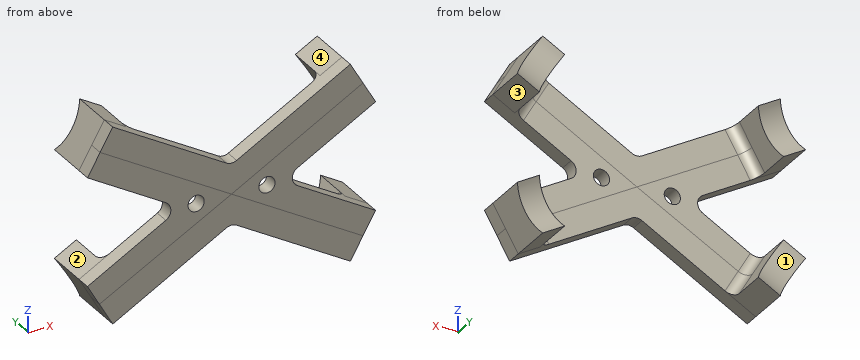
Autodesk Inventor part; units mm, degrees
ref_plane "YZ Plane" through (0, 0, 0) normal (1, 0, 0) x (0, 1, 0)
ref_plane "XZ Plane" through (0, 0, 0) normal (0, 1, 0) x (-1, 0, 0)
ref_plane "XY Plane" through (0, 0, 0) normal (0, 0, 1) x (1, 0, 0)
sketch "Sketch1" plane through (0, 0, 0) normal (0, 1, 0) x (-1, 0, 0)
  arc A0 (-1, 6.3509) -> (1, 6.3509) centre (0, 8.0829) ccw
  arc A1 (-12.9998, -1.7321) -> (-12.9998, 1.7321) centre (-13.9998, 0) ccw
  arc A2 (1, -6.3509) -> (-1, -6.3509) centre (0, -8.0829) ccw
  arc A3 (13, 1.7321) -> (13, -1.7321) centre (14, 0) ccw
  circle A4 centre (7, 0) radius 1.6
  circle A5 centre (-7, 0) radius 1.6
  line L0 (0, 0) -> (26.1212, -14.7541)
  line L1 (0, 0) -> (25.9808, 15)
  line L2 (0, 0) -> (30, 0) construction
  line L3 (0, 0) -> (-25.9808, -15)
  line L4 (0, 0) -> (-25.9808, 15)
  line L5 (0, 0) -> (30, 0) construction
  line L6 (25.9808, 15) -> (28.4808, 10.6699)
  line L7 (25.9808, 15) -> (23.4808, 19.3301)
  line L8 (1, 6.3509) -> (23.4808, 19.3301)
  line L9 (28.4808, 10.6699) -> (13, 1.7321)
  line L10 (13, -1.7321) -> (28.4808, -10.6699)
  line L11 (28.4808, -10.6699) -> (23.4808, -19.3301)
  line L12 (23.4808, -19.3301) -> (1, -6.3509)
  line L13 (-1, -6.3509) -> (-23.4808, -19.3301)
  line L14 (-23.4808, -19.3301) -> (-28.4807, -10.6699)
  line L15 (-28.4807, -10.6699) -> (-12.9998, -1.7321)
  line L16 (-12.9998, 1.7321) -> (-28.4807, 10.6699)
  line L17 (-28.4807, 10.6699) -> (-23.4808, 19.3301)
  line L18 (-23.4808, 19.3301) -> (-1, 6.3509)
  dimension "d0" = 3.2
  dimension "d1" = 30
  dimension "d2" = 30
  dimension "d3" = 30
  dimension "d4" = 30
  dimension "d5" = 30
  dimension "d6" = 150
extrude "Extrusion1" add sketch "Sketch1" along normal blind 3
sketch "Sketch2" plane through (0, 3, 0) normal (0, 1, 0) x (1, 0, 0)
  line L0 (-23.4808, -19.3301) -> (-28.4808, -10.6699)
  line L1 (-28.4808, -10.6699) -> (-24.1506, -8.1699)
  line L2 (-24.1506, -8.1699) -> (-19.1506, -16.8301)
  line L3 (-19.1506, -16.8301) -> (-23.4808, -19.3301)
  line L4 (-28.4808, -10.6699) -> (-23.4808, -19.3301)
  line L5 (-23.4808, 19.3301) -> (-28.4808, 10.6699)
  line L6 (-28.4808, 10.6699) -> (-24.1506, 8.1699)
  line L7 (-24.1506, 8.1699) -> (-19.1506, 16.8301)
  line L8 (-19.1506, 16.8301) -> (-23.4808, 19.3301)
  line L9 (-1, 6.3509) -> (-23.4808, 19.3301)
  line L10 (28.4807, 10.6699) -> (23.4808, 19.3301)
  line L11 (23.4808, 19.3301) -> (19.1506, 16.8301)
  line L12 (19.1506, 16.8301) -> (24.1506, 8.1699)
  line L13 (24.1506, 8.1699) -> (28.4807, 10.6699)
  line L14 (28.4807, -10.6699) -> (23.4808, -19.3301)
  line L15 (23.4808, -19.3301) -> (19.1506, -16.8301)
  line L16 (19.1506, -16.8301) -> (24.1506, -8.1699)
  line L17 (24.1506, -8.1699) -> (28.4807, -10.6699)
  line L18 (23.4808, -19.3301) -> (28.4807, -10.6699)
  point P0 (0, 0)
  dimension "d9" = 5
  dimension "d10" = 5
  dimension "d11" = 5
  dimension "d12" = 5
extrude "Extrusion2" add sketch "Sketch2" along normal blind 15
fillet "Fillet1" radius 2 4 edges at (-21.6506, 3, 12.5) (-21.6506, 3, -12.5) (21.6506, 3, -12.5) (21.6506, 3, 12.5)
sketch "Sketch3" plane through (-19.1506, 5, -16.8301) normal (0.866, 0, 0.5) x (0.5, 0, -0.866)
  line L0 (-10, 13) -> (0, 13)
  circle A0 centre (-5, 13) radius 8
  point P0 (-5, -5)
  dimension "d16" = 16
extrude "Extrusion3" cut sketch "Sketch3" against normal blind 13
sketch "Sketch4" plane through (23.4808, 0, -19.3301) normal (0.866, 0, -0.5) x (-0.5, 0, -0.866)
  line L0 (0, 18) -> (-9.9999, 18)
  circle A0 centre (-5, 18) radius 8
  point P0 (-5, 0)
  dimension "d19" = 16
extrude "Extrusion4" cut sketch "Sketch4" against normal blind 13
sketch "Sketch5" plane through (28.4807, 0, 10.6699) normal (0.866, 0, 0.5) x (0.5, 0, -0.866)
  line L0 (-9.9999, 18) -> (0, 18)
  circle A0 centre (-5, 18) radius 8
  point P0 (-4.9999, 0)
  dimension "d22" = 16
extrude "Extrusion5" cut sketch "Sketch5" against normal blind 10
sketch "Sketch6" plane through (-23.4808, 0, 19.3301) normal (-0.866, 0, 0.5) x (0.5, 0, 0.866)
  line L0 (0, 18) -> (-10, 18)
  circle A0 centre (-5, 18) radius 8
  point P0 (-5, 0)
  dimension "d25" = 16
extrude "Extrusion6" cut sketch "Sketch6" against normal blind 10
properties part number "Motor Support" material "ABS Plastic"
Check sheet for the modelled part. Datum: model origin and axes. Units: mm. Face numbers are marked on the shaded views. Round coordinates to 2 decimals unless told otherwise and drop trailing zeros. Write each loop counter-clockwise with the first axis right and the second up, starting at its lowest first coordinate (ties: lowest second). Pieces come first, ordered by that corner, then holes. Notation, with made-up numbers: (60.25, 9.5) -> (97.25, 9.5) arc R32 cw to (97.25, 46.5) -> close; hole circle Ø3 at (-33, -16.75). An arc over 180 degrees is marked (long way). Put each result on its own line as item: value.
(1) Sectioned sample at B-B (y = 2). Enter the section's corners in (x, z).
Values found:
outline: (-28.48, -10.67) -> (-23.48, -19.33) -> (-1, -6.35) arc R2 cw to (1, -6.35) -> (23.48, -19.33) -> (28.48, -10.67) -> (13, -1.73) arc R2 cw to (13, 1.73) -> (28.48, 10.67) -> (23.48, 19.33) -> (1, 6.35) arc R2 cw to (-1, 6.35) -> (-23.48, 19.33) -> (-28.48, 10.67) -> (-13, 1.73) arc R2 cw to (-13, -1.73) -> close; hole circle Ø3.2 at (-7, 0); hole circle Ø3.2 at (7, 0)
(2) Sectioned sample at D-D (z = 1). Enter the section's corners in (x, y).
Values found:
outline: (-12.27, 0) -> (-8.25, 0) -> (-8.25, 3) -> (-12.27, 3) -> close; (-5.75, 0) -> (5.75, 0) -> (5.75, 3) -> (-5.75, 3) -> close; (8.25, 0) -> (12.27, 0) -> (12.27, 3) -> (8.25, 3) -> close
(3) Material ranges on line 1 (X direction, y = 2, z = 0.5); line 2 (Y direction, x = -13, z = -2.5); line 3 (X direction, y = 1.5, z = -14), recorded low to high.
Values found:
line 1: x = -12.06 to -8.52, -5.48 to 5.48, 8.52 to 12.06
line 2: y = 0 to 3
line 3: x = -26.56 to -14.25, 14.25 to 26.56
(4) Go/stop test with flat-tipped pins: pin 1 Ø4.5 at (x, z) = (2, 8.5) entering from +Y; pin 2 Ø1 at (x, z) = (-20, 12.5) entering from +Y; pin 3 Ø6 at (x, y) = (-12.5, 2) entering from +Z. Record where each tip stops, or that it passes through.
Values found:
pin 1: stops at y = 3
pin 2: stops at y = 3.31
pin 3: stops at z = 14.72
(5) Sectioned sample at C-C (x = 7). Enter the section's corners in (y, z).
Values found:
outline: (0, -9.81) -> (3, -9.81) -> (3, -1.6) -> (0, -1.6) -> close; (0, 1.6) -> (3, 1.6) -> (3, 9.81) -> (0, 9.81) -> close
(6) Sectioned sample at A-A (y = 6.25). Enter the section's corners in (x, z), plus the area to 3 significant figures.
Values found:
outline: (-28.48, -10.67) -> (-23.48, -19.33) -> (-19.15, -16.83) -> (-24.15, -8.17) -> close; (-28.48, 10.67) -> (-24.15, 8.17) -> (-19.15, 16.83) -> (-23.48, 19.33) -> close; (19.15, -16.83) -> (23.48, -19.33) -> (28.48, -10.67) -> (24.15, -8.17) -> close; (19.15, 16.83) -> (24.15, 8.17) -> (28.48, 10.67) -> (23.48, 19.33) -> close
area: 200 mm^2
(7) Mould release check, pull along X, two halves, no side actions. Record for the marked faces 1, 2, 3 and 4: released by +X, released by -X, zero draft, split by the parting line, or undercut.
Values found:
face 1: undercut
face 2: released by -X
face 3: released by +X
face 4: undercut
